Part model, mm, in its own coordinate system. A direction names the side the tool comes from. Give positions to 0.01 mm unless a question says otherwise; leave off trailing zeros. Order: outer loops, then holes, each group sorted by start corner. A loop starts at its lowest first (then second) coordinate and runs counter-clockwise, first axis right, second up. Notation, with made-up numbers: (-36.75, -19) - (-0.75, -19) arc R17 cw to (-0.75, 8) - close; hole circle Ø10 at (-16.75, -4.5). An arc over 180 degrees is marked (long way). Use a Markdown table: item, result. Add a question column.
from build123d import *

# Parameters (mm, degrees)
EXTRUDE_1_DEPTH     = 14
EXTRUDE_2_DEPTH     = 2.3
SKETCH_4_R          = 2.75
EXTRUDE_3_DEPTH     = 3.5
SKETCH_5_R          = 1.7
EXTRUDE_4_DEPTH     = 6.15
FILLET_1_R          = 0.25
SKETCH_8_W          = 1
SKETCH_8_H          = 3.6
CUT_EXTRUDE_1_DEPTH = 2.75


with BuildPart() as part:
    # Эскиз1 → Бобышка-Вытянуть1 (new body)
    with BuildSketch(Plane(origin=(0, 0, 0), x_dir=(0, 0, -1), z_dir=(1, 0, 0))):
        with BuildLine():
            Line((-2.95, -1.95), (-2.95, 1.95))
            ThreePointArc((-2.95, 1.95), (0, 4.9), (2.95, 1.95))
            Line((2.95, 1.95), (2.95, -1.95))
            ThreePointArc((2.95, -1.95), (0, -4.9), (-2.95, -1.95))
        make_face()
    extrude(amount=-EXTRUDE_1_DEPTH)

    # Эскиз3 → Бобышка-Вытянуть2 (add)
    with BuildSketch(Plane.ZY.offset(14)):
        with BuildLine():
            Line((2.75, 1.95), (2.75, -1.95))
            ThreePointArc((2.75, -1.95), (0, -4.7), (-2.75, -1.95))
            Line((-2.75, -1.95), (-2.75, 1.95))
            ThreePointArc((-2.75, 1.95), (0, 4.7), (2.75, 1.95))
        make_face()
    extrude(amount=EXTRUDE_2_DEPTH)

    # Эскиз4 → Бобышка-Вытянуть3 (add)
    with BuildSketch(Plane.ZY.offset(16.3)):
        Circle(SKETCH_4_R)
    extrude(amount=EXTRUDE_3_DEPTH)

    # По траектории1: sweep along a path in Эскиз6
    with BuildLine(Plane.XY) as sweep_1_path:
        Line((-19.8, 0), (-24.776161806, 0))
        ThreePointArc((-24.776161806, 0), (-30.870449905, -0.986593903), (-36.342181829, -3.845591055))
    # Эскиз5 → По траектории1 (sweep)
    with BuildSketch(Plane.ZY.offset(19.8)):
        Circle(SKETCH_5_R)
    sweep(path=sweep_1_path.line)

    # Эскиз7 → Бобышка-Вытянуть4 (add)
    with BuildSketch(Plane(origin=(0, 0, 0), x_dir=(0, 0, -1), z_dir=(1, 0, 0))):
        Polygon((-0.05, -3.43), (-0.9, -2.58), (-0.9, 2.58), (-0.05, 3.43), (0.9, 3.43), (0.9, -3.43), align=None)
    extrude(amount=EXTRUDE_4_DEPTH)

    # Скругление1
    fillet_1_edges = [part.edges().sort_by_distance(p)[0] for p in [
        (3.075, 3.43, -0.9),
        (3.075, 3.43, 0.05),
        (3.075, 2.58, 0.9),
        (3.075, -2.58, 0.9),
        (3.075, -3.43, 0.05),
        (3.075, -3.43, -0.9),
    ]]
    fillet(fillet_1_edges, radius=FILLET_1_R)

    # Эскиз8 → Вырез-Вытянуть1 (cut)
    with BuildSketch(Plane(origin=(6.15, 0, 0), x_dir=(0, 0, -1), z_dir=(1, 0, 0))):
        with Locations((0.15, 0)):
            Rectangle(SKETCH_8_W, SKETCH_8_H)
    extrude(amount=-CUT_EXTRUDE_1_DEPTH, mode=Mode.SUBTRACT)


solid = part.part
1. Pin check, flat tips, straight feed: P1, Ø2.5, axis at x = -15.5, y = 0, coming from the +Z side; P2, Ø1, axis at x = -0.5, z = -2, coming from the +Y side; P3, Ø3, axis at x = -2.5, z = -0.5, coming from the -Y side. Stop position of each tip, or through.
2. Drill centre lines: probe 1 along Y at (x, z) = (4, -0.5); probe 2 along Z at (x, y) = (4, -1.25); probe 3 along X at (y, z) = (-0.25, -1.9). Where is each one in solid material? Low to high. Write a range as [from, to].
3. Cut at B-B (x = -9.5). Write the cut outline in (y, z).
4. Mould opens along X. For faces 4 (the face through (3, 0, 0.9)), 5 (the face through (-19.8, 0, 2)), 6 (the face through (0, 0.1, 1.3)), 7 (the face through (-18.026, -2.685, -0.596)) say: released by +X, released by -X, zero draft, split by the parting line, or undercut.
5. Tool access for faces 1 (the face through (5, 0, 0.35)), 2 (the face through (-15, 0, -2.75)), 3 (the face through (3, 0, -0.9)): list every direction of +Z, -Z, +X, -X, +Y, -Y with a clear straight run to the whole face (end or side of a thin tool).
6. Cut at A-A (y = 4). Write the cut outline in (x, z).
Responses:
| question | item | result |
|---|---|---|
| 1 | P1 | stops at z = 2.75 |
| 1 | P2 | stops at y = 4.49 |
| 1 | P3 | stops at y = -4.9 |
| 2 | probe 1 | y = [-3.43, -1.8], [1.8, 3.43] |
| 2 | probe 2 | z = [-0.9, -0.65], [0.35, 0.9] |
| 2 | probe 3 | x = [-19.8, 0] |
| 3 | outline | (-1.95, -2.95) - (1.95, -2.95) arc R2.95 ccw to (1.95, 2.95) - (-1.95, 2.95) arc R2.95 ccw to start |
| 4 | face 4 | zero draft |
| 4 | face 5 | undercut |
| 4 | face 6 | released by +X |
| 4 | face 7 | undercut |
| 5 | face 1 | +X |
| 5 | face 2 | -Z, -X, +Y, -Y |
| 5 | face 3 | -Z, +X, +Y, -Y |
| 6 | outline | (-16.3, -1.83) - (-14, -1.83) - (-14, -2.12) - (0, -2.12) - (0, 2.12) - (-14, 2.12) - (-14, 1.83) - (-16.3, 1.83) - close |
